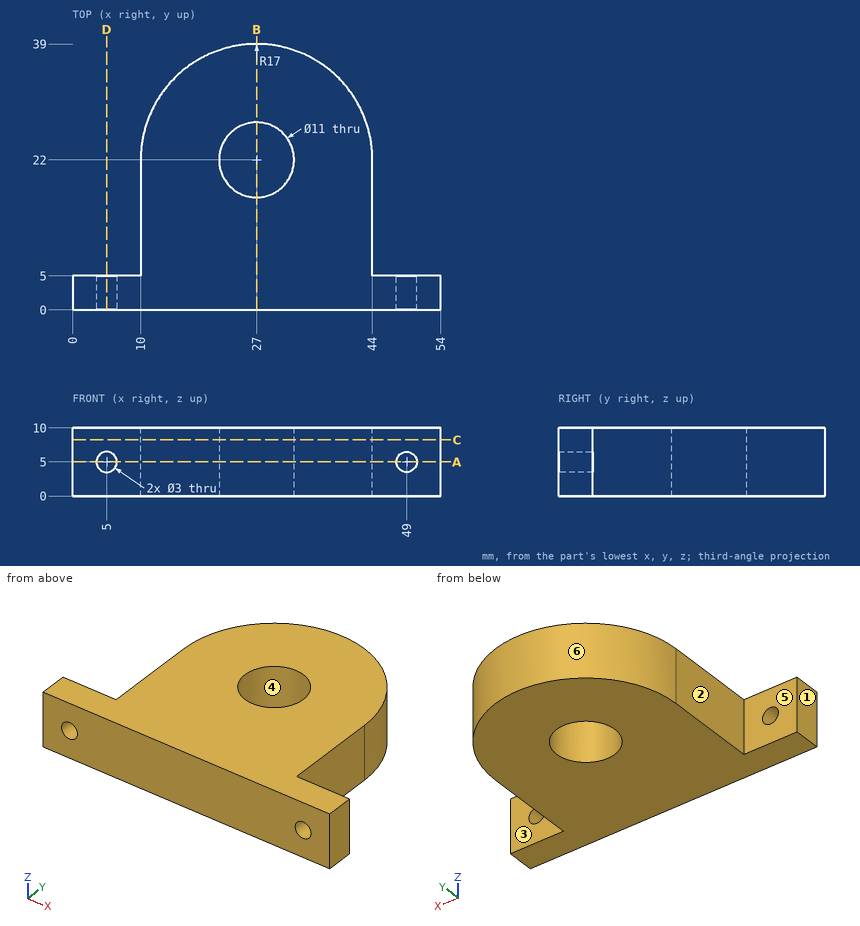
Geometry check sheet. Reference: drawing and pictorial views, mm from the part's lowest x, y, z. A direction names the side the tool comes from. Give positions to 0.01 mm unless a question says otherwise; leave off trailing zeros. Loops run counter-clockwise (first coordinate to the right, second up) from the corner with the lowest first, then second, coordinate; pieces in that order, holes last. Notation, with made-up numbers: M 64,24 L 83,24 A24 ccw 83,40 Z; hole C 47.5,76 d6. An arc over 180 degrees is marked long. Use a Markdown table: item, result. Add a question column.
Q1. Sectioned sample at C-C, the plane z = 8.25. Record the cut outline in (x, y).
Q2. Sectioned sample at D-D, the plane x = 5. Record the cut outline in (y, z).
Q3. Scan lines: line 1 along X through (y, z) = (3.5, 5); line 2 along Z through (x, y) = (5, 2); line 3 along X through (y, z) = (2, 4). Record each from-to range of solid material in increasing order. Write a range as [from, to].
Q4. Mould release check, pull along X, two halves, no side actions. Record for the marked faces 4, 5 and 6: pulls with the +X half, pulls with the -X half, needs draft (parallel to the pull), parting line crosses it, or undercut.
Q5. Go/stop test with flat-tipped pins: pin 1 (2.5 mm diameter, centred on x = 5, z = 5, fed in from +Y); pin 2 (6 mm diameter, centred on y = 5, z = 4, fed in from -X); pin 3 (1.5 mm diameter, centred on y = 23, z = 7, fed in from -X); pin 4 (3 mm diameter, centred on x = 38.5, z = 4, fed in from +Y). Record where each tip stops, or that it passes through.
Q6. Sectioned sample at B-B, the plane x = 27. Record the cut outline in (y, z).
Q7. Sectioned sample at A-A, the plane z = 5. Record the cut outline in (x, y).
Q8. Tool access check on the marked faces 1, 2 and 3. Record the directions out of +Z, -Z, +X, -X, +Y, -Y that give a thin tool (end or side, any length) a straight path to the whole face; none if there is none.
Verdict:
| question | item | result |
|---|---|---|
| 1 | outline | M 0,0 L 54,0 L 54,5 L 44,5 L 44,22 A17 ccw 10,22 L 10,5 L 0,5 Z; hole C 27,22 d11 |
| 2 | outline | M 0,0 L 5,0 L 5,3.5 L 0,3.5 Z; M 0,6.5 L 5,6.5 L 5,10 L 0,10 Z |
| 3 | line 1 | [0, 3.5], [6.5, 47.5], [50.5, 54] |
| 3 | line 2 | [0, 3.5], [6.5, 10] |
| 3 | line 3 | [0, 3.88], [6.12, 47.88], [50.12, 54] |
| 4 | face 4 | undercut |
| 4 | face 5 | needs draft |
| 4 | face 6 | parting line crosses it |
| 5 | pin 1 | through |
| 5 | pin 2 | x = 0 |
| 5 | pin 3 | x = 10 |
| 5 | pin 4 | y = 35.75 |
| 6 | outline | M 0,0 L 16.5,0 L 16.5,10 L 0,10 Z; M 27.5,0 L 39,0 L 39,10 L 27.5,10 Z |
| 7 | outline | M 0,0 L 3.5,0 L 3.5,5 L 0,5 Z; M 6.5,0 L 47.5,0 L 47.5,5 L 44,5 L 44,22 A17 ccw 10,22 L 10,5 L 6.5,5 Z; M 50.5,0 L 54,0 L 54,5 L 50.5,5 Z; hole C 27,22 d11 |
| 8 | face 1 | +Z, -Z, -X, +Y, -Y |
| 8 | face 2 | +Z, -Z, -X, +Y |
| 8 | face 3 | +Z, -Z, +X, +Y |
